Drawing for the job (mm, zero at the part's lowest x, y, z). Round coordinates to 2 decimals unless told otherwise and drop trailing zeros. One line per question, with ' | ' between items.
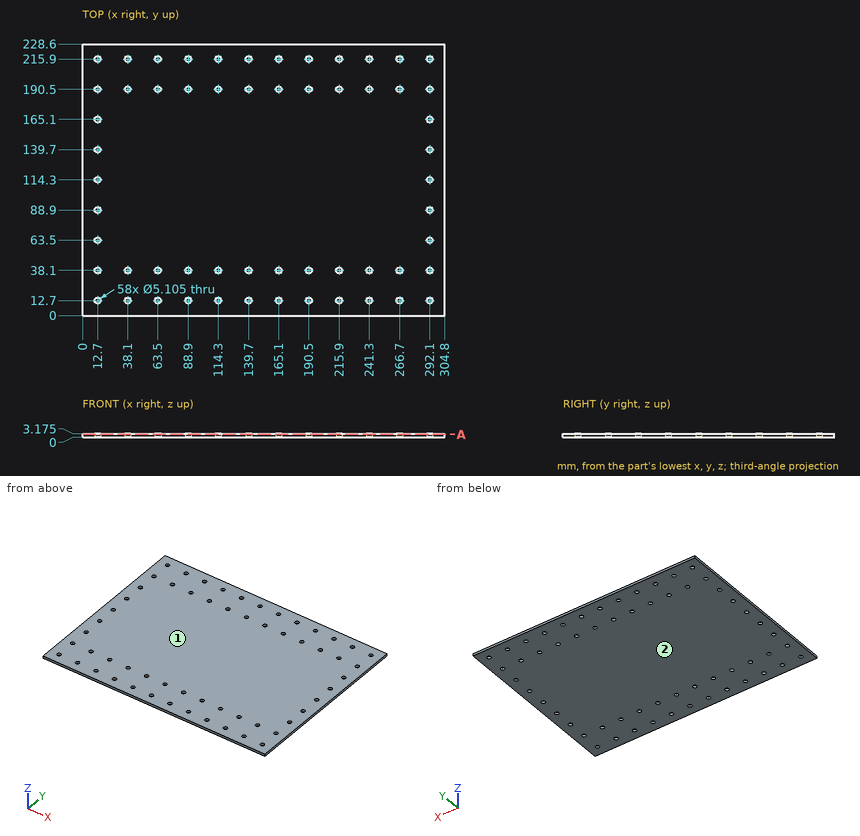
(1) Drop flat-ended pins along their axis: pin 1 (6 mm diameter, centred on x = 114.3, y = 190.5, fed in from -Z); pin 2 (4.5 mm diameter, centred on x = 165.1, y = 12.7, fed in from +Z). Give the stop position or say it passes through.
Calculated:
pin 1: z = 0 | pin 2: through
(2) Slice it at A-A (z = 2.6). State how many separate pieces and enclosed holes the cut face has, then the cut area to 3 significant figures.
Calculated:
separate pieces: 1 | enclosed holes: 58 | area: 68,500 mm2
(3) Mould opens along Z. For the marked faces 1 and 2 say: pulls with the +Z half, pulls with the -Z half, needs draft (parallel to the pull), parting line crosses it, or undercut.
Calculated:
face 1: pulls with the +Z half | face 2: pulls with the -Z half
(4) Wall check: line 1 (Y direction, x = 63.5, z = 1.1); line 2 (X direction, y = 165.1, z = 1.2); line 3 (X direction, y = 63, z = 0.7). Give the ranges that are in metal, low to high. Write a range as from..to.
Calculated:
line 1: 0..10.15, 15.25..35.55, 40.65..187.95, 193.05..213.35, 218.45..228.6 | line 2: 0..10.15, 15.25..289.55, 294.65..304.8 | line 3: 0..10.2, 15.2..289.6, 294.6..304.8
